```python
from build123d import *

# Parameters (mm, degrees)
SKETCH9_W               = 15
SKETCH9_H               = 8.35
BOSS_EXTRUDE4_DEPTH     = 50
CUT_EXTRUDE4_DEPTH      = 23.76
BOSS_EXTRUDE9_DEPTH     = 15
CUT_EXTRUDE5_REACH      = 31.734
SKETCH10_R              = 2.7
SKETCH12_W              = 3
SKETCH12_H              = 3
BOSS_EXTRUDE5_DEPTH     = 5
SKETCH13_W              = 2
SKETCH13_H              = 3
CUT_EXTRUDE6_DEPTH      = 1
BOSS_EXTRUDE6_DEPTH     = 3
SKETCH22_W              = 2
SKETCH22_H              = 2
BOSS_EXTRUDE10_DEPTH    = 15
CUT_EXTRUDE7_REACH      = 55.801
CUT_EXTRUDE7_END_RADIUS = 2.7
SKETCH23_R              = 2.5
SKETCH24_W              = 2
SKETCH24_H              = 5
BOSS_EXTRUDE11_DEPTH    = 5
BOSS_EXTRUDE12_DEPTH    = 15


with BuildPart() as part:
    # Sketch9 → Boss-Extrude4 (new body)
    with BuildSketch(Plane.XY):
        with Locations((0, 4.175)):
            Rectangle(SKETCH9_W, SKETCH9_H)
    extrude(amount=BOSS_EXTRUDE4_DEPTH)

    # Sketch7 → Cut-Extrude4 (cut)
    with BuildSketch(Plane.XY):
        Polygon((-5.5, 2), (-5.5, 4.8), (-2.75, 4.8), (-2.75, 8.35), (2.75, 8.35), (2.75, 4.8), (5.5, 4.8), (5.5, 2), align=None)
    extrude(amount=CUT_EXTRUDE4_DEPTH, mode=Mode.SUBTRACT)

    # Sketch21 → Boss-Extrude9 (add)
    with BuildSketch(Plane.ZY.offset(7.5)):
        Polygon((50, 0), (51.294730508, 0), (50, 8.35), align=None)
    extrude(amount=-BOSS_EXTRUDE9_DEPTH)

    # Cut-Extrude5: up to this plane
    cut_extrude5_end = Plane(origin=(15.949782665, 0, 51.294730508), z_dir=(0, 0.15322648630316937, 0.9881910968507989))
    # Sketch10 → Cut-Extrude5 (cut, up to the surface)
    with BuildSketch(Plane.XY.offset(23.76), mode=Mode.PRIVATE) as cut_extrude5_sk1:
        with Locations(Location((0, 4.7, 0), (0, 0, 270))):
            Circle(SKETCH10_R)
    cut_extrude5_tool1 = split(extrude(cut_extrude5_sk1.sketch, amount=CUT_EXTRUDE5_REACH, mode=Mode.PRIVATE), bisect_by=cut_extrude5_end, keep=Keep.BOTH, mode=Mode.PRIVATE)
    add(cut_extrude5_tool1.solids().sort_by_distance((0, 4.7, 23.76))[0], mode=Mode.SUBTRACT)

    # Sketch12 → Boss-Extrude5 (add)
    with BuildSketch(Plane(origin=(7.5, 0, 0), x_dir=(0, 0, -1), z_dir=(1, 0, 0))):
        with Locations((-45.5, 3.64)):
            Rectangle(SKETCH12_W, SKETCH12_H)
    boss_extrude5 = extrude(amount=BOSS_EXTRUDE5_DEPTH)

    # Sketch13 → Cut-Extrude6 (cut)
    with BuildSketch(Plane.XY.offset(47)):
        with Locations((10, 3.64)):
            Rectangle(SKETCH13_W, SKETCH13_H)
    cut_extrude6 = extrude(amount=-CUT_EXTRUDE6_DEPTH, mode=Mode.SUBTRACT)

    # Mirror2: Boss-Extrude5 across plane
    add(boss_extrude5.mirror(Plane(origin=(0, 0, 0), x_dir=(0, 0, 1), z_dir=(1, 0, 0))))

    # Mirror4: Cut-Extrude6 across plane
    add(cut_extrude6.mirror(Plane(origin=(0, 0, 0), x_dir=(0, 0, 1), z_dir=(1, 0, 0))), mode=Mode.SUBTRACT)

    # Sketch14 → Boss-Extrude6 (add)
    with BuildSketch(Plane(origin=(0, 5.14, 0), x_dir=(1, 0, 0), z_dir=(0, 1, 0))):
        Polygon((12.5, -44), (7.5, -40), (7.5, -44), align=None)
    boss_extrude6 = extrude(amount=-BOSS_EXTRUDE6_DEPTH)

    # Mirror5: Boss-Extrude6 across plane
    add(boss_extrude6.mirror(Plane(origin=(0, 0, 0), x_dir=(0, 0, 1), z_dir=(1, 0, 0))))

    # Sketch22 → Boss-Extrude10 (add)
    with BuildSketch(Plane.ZY.offset(7.5)):
        with Locations((47.655054804, -1)):
            Rectangle(SKETCH22_W, SKETCH22_H)
        with Locations((47.655054804, 9.35)):
            Rectangle(SKETCH22_W, SKETCH22_H)
    extrude(amount=-BOSS_EXTRUDE10_DEPTH)

    # Cut-Extrude7: up to this cylinder (the profile starts outside it)
    cut_extrude7_end = Plane(origin=(0, 4.7, 29.26), z_dir=(0, 0, -1)) * Cylinder(CUT_EXTRUDE7_END_RADIUS, 118.002, mode=Mode.PRIVATE)
    # Sketch23 → Cut-Extrude7 (cut, up to the surface)
    with BuildSketch(Plane.XZ, mode=Mode.PRIVATE) as cut_extrude7_sk1:
        with Locations(Location((0, 29.26, 0), (0, 0, 270))):
            Circle(SKETCH23_R)
    cut_extrude7_tool1 = extrude(cut_extrude7_sk1.sketch, amount=-CUT_EXTRUDE7_REACH, mode=Mode.PRIVATE) - cut_extrude7_end
    add(cut_extrude7_tool1.solids().sort_by_distance((0, 0, 29.26))[0], mode=Mode.SUBTRACT)

    # Sketch24 → Boss-Extrude11 (add)
    with BuildSketch(Plane.XZ):
        with Locations((6.5, 33.76)):
            Rectangle(SKETCH24_W, SKETCH24_H)
        with Locations((-6.5, 33.76)):
            Rectangle(SKETCH24_W, SKETCH24_H)
        with BuildLine():
            Line((2.5, 33.01), (-2.5, 33.01))
            ThreePointArc((-2.5, 33.01), (-3.25, 33.76), (-2.5, 34.51))
            Line((-2.5, 34.51), (2.5, 34.51))
            ThreePointArc((2.5, 34.51), (3.25, 33.76), (2.5, 33.01))
        make_face()
    extrude(amount=BOSS_EXTRUDE11_DEPTH)

    # Sketch25 → Boss-Extrude12 (add)
    with BuildSketch(Plane(origin=(7.5, 0, 0), x_dir=(0, 0, -1), z_dir=(1, 0, 0))):
        Polygon((-30.558938802, 8.35), (-36.961061198, 8.35), (-36.961061198, 16.922552294), (-30.558938802, 17.980397342), align=None)
    extrude(amount=-BOSS_EXTRUDE12_DEPTH)


solid = part.part
```
Here's how the part is built. I have some questions about the finished solid (model axes, mm). A direction names the side the tool comes from. Coordinates: 2 decimals unless noted, no trailing zeros. Loops run counter-clockwise (first coordinate to the right, second up) from the corner with the lowest first, then second, coordinate; pieces in that order, holes last. Notation, with made-up numbers: M 6,-23 L 46,-23 A30 ccw 46,7 Z; hole C 4,-17.5 d6. An arc over 180 degrees is marked long. One line per item, written item: value.
1. Imagine slicing it at C-C (z = 29.26). List the corners of the cut face in (x, y) for me, and give its area (3 significant figures).
Geometry says:
outline: M -7.5,0 L -2.5,0 L -2.5,3.68 A2.7 cw long 2.5,3.68 L 2.5,0 L 7.5,0 L 7.5,8.35 L -7.5,8.35 Z
area: 90.0 mm2
2. Imagine slicing it at D-D (y = 6.75). List the corners of the cut face in (x, z) for me, and give its area (3 significant figures).
Geometry says:
outline: M -7.5,0 L -2.75,0 L -2.75,23.76 L -1.76,23.76 L -1.76,50.25 L -7.5,50.25 Z; M 1.76,23.76 L 2.75,23.76 L 2.75,0 L 7.5,0 L 7.5,50.25 L 1.76,50.25 Z
area: 530 mm2
3. Will these pins go through, and if not, where does the flat tip stop? pin 1 Ø1.6 at (x, z) = (-2, 47.5) entering from +Y; pin 2 Ø2 at (x, y) = (-7, -1.5) entering from -Z; pin 3 Ø1 at (x, y) = (5, 14.5) entering from -Z; pin 4 Ø12 at (x, y) = (8, -0.5) entering from +Z.
Geometry says:
pin 1: stops at y = 10.35
pin 2: stops at z = 31.26
pin 3: stops at z = 30.56
pin 4: stops at z = 51.29
4. Thinking about a two-plate mould opening in X: for faces 4 (the cylindrical face through (-3.25, -2.46, 33.74)), 5 (the flat face through (-12, 4, 47)), 6 (the flat face through (-12.5, 4, 46)), which applies, +X half, -X half, draft (parallel to the pull), parting line (faces both ways), or undercut?
Geometry says:
face 4: undercut
face 5: draft
face 6: -X half
5. Imagine slicing it at A-A (z = 47.5). List the corners of the cut face in (x, y) for me, and give its area (3 significant figures).
Geometry says:
outline: M -7.5,-2 L 7.5,-2 L 7.5,10.35 L -7.5,10.35 Z; hole C 0,4.7 d5.4
area: 162 mm2
6. Please list where these lines run through material, in increasing order: probe 1 along X at (y, z) = (2.45, 29.26); probe 2 along X at (y, z) = (4.7, 38.5); probe 3 along Y at (x, z) = (-1, 39.5).
Geometry says:
probe 1: x = -7.5 to -2.5, 2.5 to 7.5
probe 2: x = -7.5 to -2.7, 2.7 to 7.5
probe 3: y = 0 to 2.19, 7.21 to 8.35
7. Imagine slicing it at B-B (x = -1). State how many separate pieces and enclosed holes the cut face has, and give its area (3 significant figures).
Geometry says:
separate pieces: 3
enclosed holes: 0
area: 201 mm2
8. On a 3-axis mill with a long thin cutter (end or side, diameter ignored), from which of +Z, -Z, +X, -X, +Y, -Y can I reach the whole of each face in a straight line? I mean faces 1 (the flat face through (12, 4, 47)), 2 (the flat face through (0, -2, 33.01)), 3 (the flat face through (-11, 3.6, 46.5)). Say none if no direction works.
Geometry says:
face 1: +Z, +X, +Y, -Y
face 2: -Z, -Y
face 3: +Z, +Y, -Y
